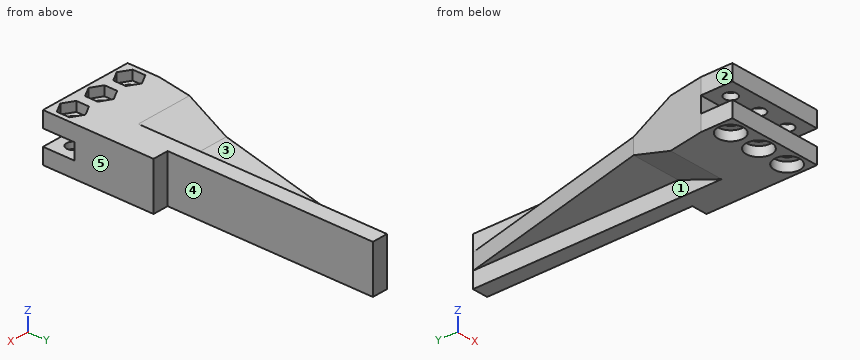
from build123d import *

# Parameters (mm, degrees)
SKETCH1_W                                        = 10
SKETCH1_H                                        = 65
SKETCH1_H_2                                      = 25
SKETCH1_W_2                                      = 5
SKETCH1_H_3                                      = 10
SKETCH1_W_3                                      = 15
BOSS_EXTRUDE1_DEPTH                              = 15
CBORE_FOR_M4_HEX_HEAD_MACHINE_SCREW1_D           = 4
CBORE_FOR_M4_HEX_HEAD_MACHINE_SCREW1_CBORE_D     = 8
CBORE_FOR_M4_HEX_HEAD_MACHINE_SCREW1_CBORE_DEPTH = 3
CUT_EXTRUDE1_DEPTH                               = 3
SKETCH7_W                                        = 5
SKETCH7_H                                        = 10
CUT_EXTRUDE2_DEPTH                               = 106.475115549
CUT_EXTRUDE3_DEPTH                               = 106.475115549
CUT_EXTRUDE4_DEPTH                               = 5
CUT_EXTRUDE5_DEPTH                               = 5
CHAMFER1_SIZE2                                   = 5
CHAMFER1_SIZE                                    = 13.737387097
CHAMFER2_SIZE2                                   = 5
CHAMFER2_SIZE                                    = 13.737387097


with BuildPart() as part:
    # Sketch1 → Boss-Extrude1 (new body)
    with BuildSketch(Plane.XY):
        Polygon((-30, 10), (-15, 10), (-15, 35), (-15, 100), align=None)
        with Locations((-10, 67.5)):
            Rectangle(SKETCH1_W, SKETCH1_H)
        with Locations((-10, 22.5)):
            Rectangle(SKETCH1_W, SKETCH1_H_2)
        with Locations((-2.5, 22.5)):
            Rectangle(SKETCH1_W_2, SKETCH1_H_2)
        with Locations((-2.5, 5)):
            Rectangle(SKETCH1_W_2, SKETCH1_H_3)
        with Locations((-10, 5)):
            Rectangle(SKETCH1_W, SKETCH1_H_3)
        with Locations((-22.5, 5)):
            Rectangle(SKETCH1_W_3, SKETCH1_H_3)
    extrude(amount=BOSS_EXTRUDE1_DEPTH)

    # CBORE for M4 Hex Head Machine Screw1 (through all)
    with Locations(Plane(origin=(0, 0, 0), x_dir=(-1, 0, 0), z_dir=(0, 0, -1))):
        with Locations((25, 5), (15, 5), (5, 5)):
            CounterBoreHole(CBORE_FOR_M4_HEX_HEAD_MACHINE_SCREW1_D / 2, CBORE_FOR_M4_HEX_HEAD_MACHINE_SCREW1_CBORE_D / 2, CBORE_FOR_M4_HEX_HEAD_MACHINE_SCREW1_CBORE_DEPTH)

    # Sketch6 → Cut-Extrude1 (cut)
    with BuildSketch(Plane.XY.offset(15)):
        Polygon((-15, 9), (-18.464101615, 7), (-18.464101615, 3), (-15, 1), (-11.535898385, 3), (-11.535898385, 7), align=None)
        Polygon((-25, 9), (-28.464101615, 7), (-28.464101615, 3), (-25, 1), (-21.535898385, 3), (-21.535898385, 7), align=None)
        Polygon((-5, 9), (-8.464101615, 7), (-8.464101615, 3), (-5, 1), (-1.535898385, 3), (-1.535898385, 7), align=None)
    extrude(amount=-CUT_EXTRUDE1_DEPTH, mode=Mode.SUBTRACT)

    # Sketch7 → Cut-Extrude2 (cut, through all)
    with BuildSketch(Plane.ZY.offset(30)):
        with Locations((7.5, 5)):
            Rectangle(SKETCH7_W, SKETCH7_H)
    extrude(amount=-CUT_EXTRUDE2_DEPTH, mode=Mode.SUBTRACT)

    # Sketch8 → Cut-Extrude3 (cut, through all)
    with BuildSketch(Plane(origin=(0, 0, 0), x_dir=(-1, 0, 0), z_dir=(0, 0, -1))):
        Polygon((15, 100), (10, 100), (25.833333333, 35), align=None)
    extrude(amount=-CUT_EXTRUDE3_DEPTH, mode=Mode.SUBTRACT)

    # Sketch9 → Cut-Extrude4 (cut)
    with BuildSketch(Plane(origin=(0, 0, 0), x_dir=(-1, 0, 0), z_dir=(0, 0, -1))):
        Polygon((10, 100), (10, 35), (25.833333333, 35), align=None)
    extrude(amount=-CUT_EXTRUDE4_DEPTH, mode=Mode.SUBTRACT)

    # Sketch10 → Cut-Extrude5 (cut)
    with BuildSketch(Plane.XY.offset(15)):
        Polygon((-10, 100), (-10, 35), (-25.833333333, 35), align=None)
    extrude(amount=-CUT_EXTRUDE5_DEPTH, mode=Mode.SUBTRACT)

    # Chamfer1
    chamfer1_edges = [part.edges().sort_by_distance(p)[0] for p in [
        (-17.916666667, 35, 15),
    ]]
    chamfer1_side = [part.faces().sort_by_distance(p)[0] for p in [
        (-17.916666667, 34.9, 15),
    ]]
    chamfer(chamfer1_edges, length=CHAMFER1_SIZE - 0.0001, length2=CHAMFER1_SIZE2 - 0.0001, reference=chamfer1_side[0])  # a hair under: the kernel refuses the full size

    # Chamfer2
    chamfer2_edges = [part.edges().sort_by_distance(p)[0] for p in [
        (-17.916666667, 35, 0),
    ]]
    chamfer2_side = [part.faces().sort_by_distance(p)[0] for p in [
        (-17.916666667, 34.9, 0),
    ]]
    chamfer(chamfer2_edges, length=CHAMFER2_SIZE - 0.0001, length2=CHAMFER2_SIZE2 - 0.0001, reference=chamfer2_side[0])  # a hair under: the kernel refuses the full size


solid = part.part
Can you work these out from the model? Positions are in its coordinate system, mm. Face numbers are marked on the shaded views. A direction names the side the tool comes from. Coordinates: 2 decimals unless noted, no trailing zeros. Loops run counter-clockwise (first coordinate to the right, second up) from the corner with the lowest first, then second, coordinate; pieces in that order, holes last. Notation, with made-up numbers: M -7,20 L 46,20 A27 cw 46,48 Z; hole C 68.5,61.25 d11. An arc over 180 degrees is marked long. Return JSON: item names as keys, results as strings. Group by question number.
Item 1: On a 3-axis mill with a long thin cutter (end or side, diameter ignored), from which of +Z, -Z, +X, -X, +Y, -Y can I reach the whole of each face in a straight line? I mean the marked faces 1, 2, 3, 4 and 5. Say none if no direction works.
Item 2: Imagine slicing it at B-B (y = 70.5). Please give me the cut outline in (x, z).
Item 3: Imagine slicing it at C-C (y = 5). Give the number of separate pieces and of enclosed holes in the cut face, and give its area (3 significant figures).
Item 4: If I drill on L1, parallel to Z at x = -12.5, y = 5.5; L2, parallel to Z at x = -25.75, y = 9.5; L3, parallel to Z at x = -18.5, y = 62.5, over which ranges is the centre line in solid material (lowest first)? Write a range as from..to.
Item 5: Imagine slicing it at D-D (y = 59.5). Please give me the cut outline in (x, z), and give its area (3 significant figures).
Item 6: I'm going to push flat-ended pins straight in: pin 1 Ø2.5 at (y, z) = (77.5, 2) entering from -X; pin 2 Ø2.5 at (x, y) = (-14.5, 6.5) entering from -Z; pin 3 Ø1 at (y, z) = (23, 13.5) entering from -X. Where does each tip first touch, or does it pass through?
Verdict:
{
 "1": {"face 1": "-Z, -X, +Y", "face 2": "+Z, -Z, -X, +Y, -Y", "face 3": "+Z, -X, +Y", "face 4": "+Z, -Z, +X, +Y", "face 5": "+Z, -Z, +X, +Y, -Y"},
 "2": {"outline": "M -17.19,5 L -10,5 L -10,0 L -5,0 L -5,15 L -10,15 L -10,10 L -17.19,10 Z"},
 "3": {"separate pieces": "8", "enclosed holes": "0", "area": "118 mm^2"},
 "4": {"L1": "z = 3..5, 10..12", "L2": "z = 0..5, 10..15", "L3": "z = 5..10"},
 "5": {"outline": "M -19.87,5 L -10,5 L -10,0 L -5,0 L -5,15 L -10,15 L -10,10 L -19.87,10 Z", "area": "124 mm^2"},
 "6": {"pin 1": "stops at x = -10", "pin 2": "stops at z = 3", "pin 3": "stops at x = -27.92"}
}
